Here's the drawing with two shaded views (mm, measured from the low corner). I have some questions. A direction names the side the tool comes from. Coordinates: 2 decimals unless noted, no trailing zeros. Write each loop counter-clockwise with the first axis right and the second up, starting at its lowest first coordinate (ties: lowest second). Pieces come first, ordered by that corner, then holes. Notation, with made-up numbers: M 7,42.25 L 17,42.25 A22 ccw 17,66.25 Z; hole C -29.5,10 d11. An arc over 180 degrees is marked long. Use one line per item in the form item = value. Start each with the question number.
1. I want a section at D-D, the plane z = 28. List the corners of the cut face in (x, y) for me.
2. On a 3-axis mill with a long thin cutter (end or side, diameter ignored), from which of +Z, -Z, +X, -X, +Y, -Y can I reach the whole of each face in a straight line? I mean the marked faces 5 and 6. Say none if no direction works.
3. I want a section at A-A, the plane y = 5. List the corners of the cut face in (x, z) for me.
4. Thinking about a two-plate mould opening in Y: for the marked faces 1, 2, 3 and 4, which applies, released by +Y, released by -Y, zero draft, split by the parting line, or undercut?
5. I want a section at C-C, the plane z = 4. List the corners of the cut face in (x, y) for me, plus the area to 3 significant figures.
6. I'm going to push flat-ended pins straight in: pin 1 Ø3 at (x, z) = (2.5, 22) entering from -Y; pin 2 Ø2.5 at (x, y) = (4.5, 0.5) entering from +Z; pin 3 Ø3 at (y, z) = (3.175, 3.175) entering from -X; pin 4 Ø1.9 at (x, z) = (3.5, 17) entering from +Y. Where does each tip first touch, or does it pass through?
7. Please list where these lines run through material, in increasing order: line 1 along Z through (x, y) = (4.75, 3.25); line 2 along Y through (x, z) = (3, 22); line 3 along Z through (x, y) = (1, 4). Write a range as [from, to].
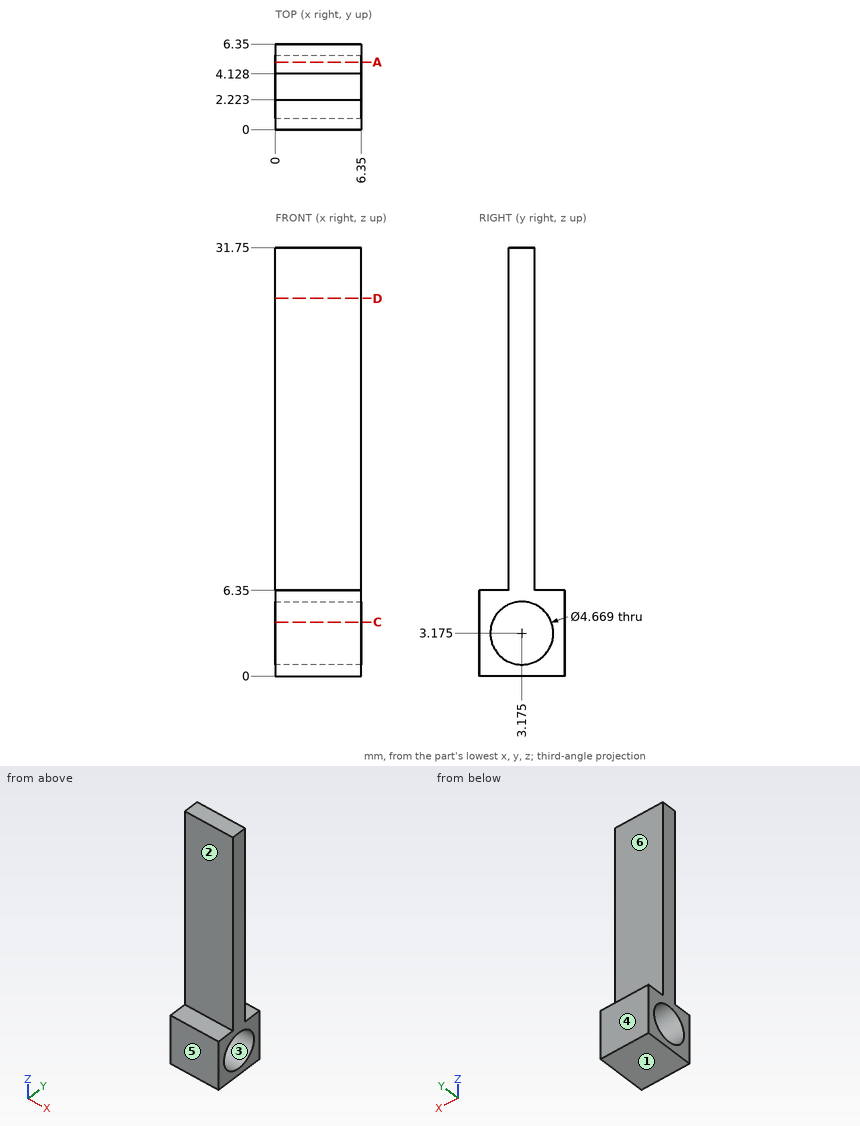
Answer list:
q1.outline = M 0,2.22 L 6.35,2.22 L 6.35,4.13 L 0,4.13 Z
q2.face_5 = +Z, -Z, +X, -X, -Y
q2.face_6 = +Z, +X, -X, +Y
q3.outline = M 0,0 L 6.35,0 L 6.35,1.72 L 0,1.72 Z; M 0,4.63 L 6.35,4.63 L 6.35,6.35 L 0,6.35 Z
q4.face_1 = zero draft
q4.face_2 = released by -Y
q4.face_3 = undercut
q4.face_4 = released by +Y
q5.outline = M 0,0 L 6.35,0 L 6.35,0.99 L 0,0.99 Z; M 0,5.36 L 6.35,5.36 L 6.35,6.35 L 0,6.35 Z
q5.area = 12.6 mm²
q6.pin_1 = 2.22
q6.pin_2 = 6.35
q6.pin_3 = through
q6.pin_4 = 4.13
q7.line_1 = [0, 0.84], [5.51, 31.75]
q7.line_2 = [2.22, 4.13]
q7.line_3 = [0, 0.99], [5.36, 31.75]
